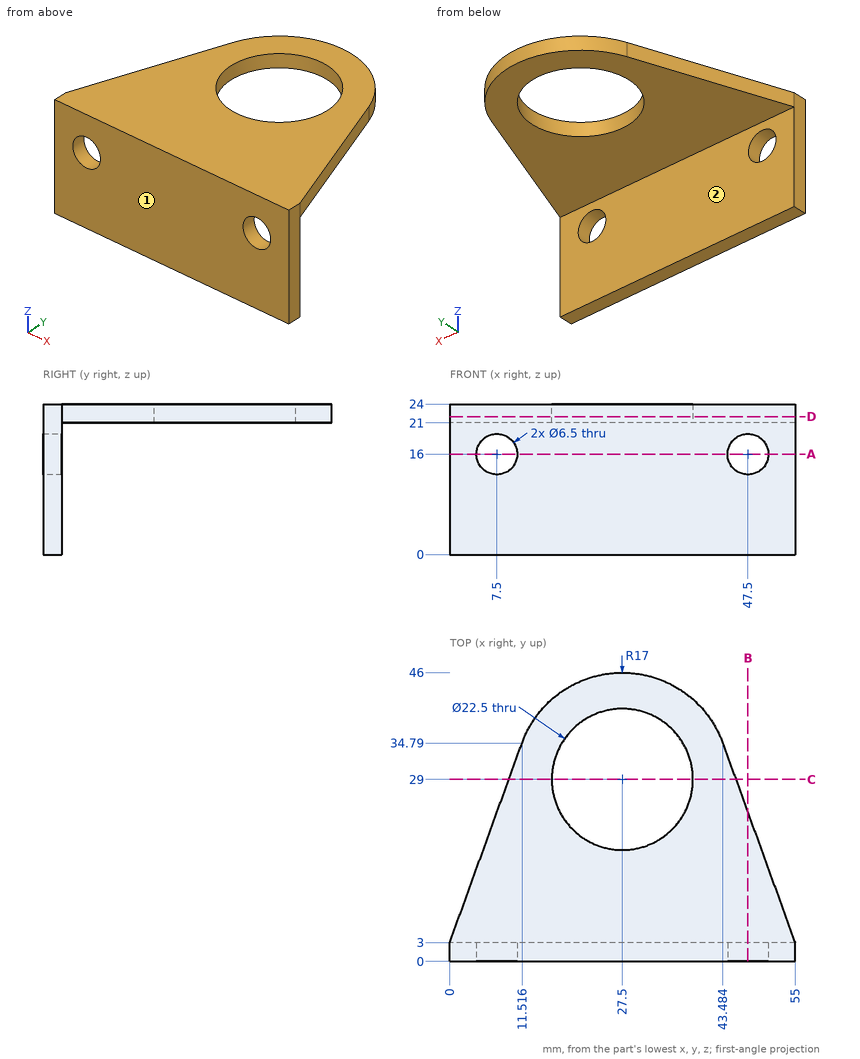
Geometry check sheet. Reference: drawing and pictorial views, mm from the part's lowest x, y, z. A direction names the side the tool comes from. Coordinates: 2 decimals unless noted, no trailing zeros. Loops run counter-clockwise (first coordinate to the right, second up) from the corner with the lowest first, then second, coordinate; pieces in that order, holes last. Notation, with made-up numbers: (63.5, -25.75) -> (77.5, -25.75) arc R16 cw to (77.5, 2.25) -> close; hole circle Ø8 at (27.25, -16.5). An arc over 180 degrees is marked (long way). Write item = value, one per line. Start each with the question number.
1. Section check A-A on z = 16. Record the cut outline in (x, y).
2. Depth check by flat-ended pin: P1, Ø1, axis at x = 35.5, z = 6.5, coming from the -Y side; P2, Ø6.5, axis at x = 39, z = 9.5, coming from the +Y side; P3, Ø10, axis at x = 48.5, y = 13.5, coming from the -Z side. Enter the tip coordinate at first touch or a pass-through.
3. Section check B-B on x = 47.5. Record the cut outline in (y, z), then the cut area to 3 significant figures.
4. Material ranges on line 1 (X direction, y = 1.15, z = 16); line 2 (Y direction, x = 37.5, z = 19.25); line 3 (Z direction, x = 31, y = 42), recorded low to high.
5. Tool access check on the marked faces 1 and 2. Record the directions out of +Z, -Z, +X, -X, +Y, -Y that give a thin tool (end or side, any length) a straight path to the whole face; none if there is none.
6. Section check C-C on y = 29. Record the cut outline in (x, z).
7. Section check D-D on z = 22. Record the cut outline in (x, y).
Responses:
q1.outline = (0, 0) -> (4.25, 0) -> (4.25, 3) -> (0, 3) -> close; (10.75, 0) -> (44.25, 0) -> (44.25, 3) -> (10.75, 3) -> close; (50.75, 0) -> (55, 0) -> (55, 3) -> (50.75, 3) -> close
q2.P1 = 0
q2.P2 = 3
q2.P3 = 21
q3.outline = (0, 0) -> (3, 0) -> (3, 12.75) -> (0, 12.75) -> close; (0, 19.25) -> (3, 19.25) -> (3, 21) -> (23.7, 21) -> (23.7, 24) -> (0, 24) -> close
q3.area = 115 mm2
q4.line_1 = 0 to 4.25, 10.75 to 44.25, 50.75 to 55
q4.line_2 = 0 to 3
q4.line_3 = 21 to 24
q5.face_1 = +Z, -Z, +X, -X, -Y
q5.face_2 = -Z, +X, -X, +Y
q6.outline = (9.42, 21) -> (16.25, 21) -> (16.25, 24) -> (9.42, 24) -> close; (38.75, 21) -> (45.58, 21) -> (45.58, 24) -> (38.75, 24) -> close
q7.outline = (0, 0) -> (55, 0) -> (55, 3) -> (43.48, 34.79) arc R17 ccw to (11.52, 34.79) -> (0, 3) -> close; hole circle Ø22.5 at (27.5, 29)
